Can you work these out from the drawing? Everything is in mm from the part's minimum corner. A direction names the side the tool comes from. Coordinates: 2 decimals unless noted, no trailing zeros. Loops run counter-clockwise (first coordinate to the right, second up) from the corner with the lowest first, then second, coordinate; pieces in that order, holes last. Notation, with made-up numbers: (50.25, -4.5) - (102.25, -4.5) arc R22 cw to (102.25, 25.5) - close; hole circle Ø10 at (55.5, 17). An arc over 180 degrees is marked (long way). Put each result on its own line as item: value. Start each with the question number.
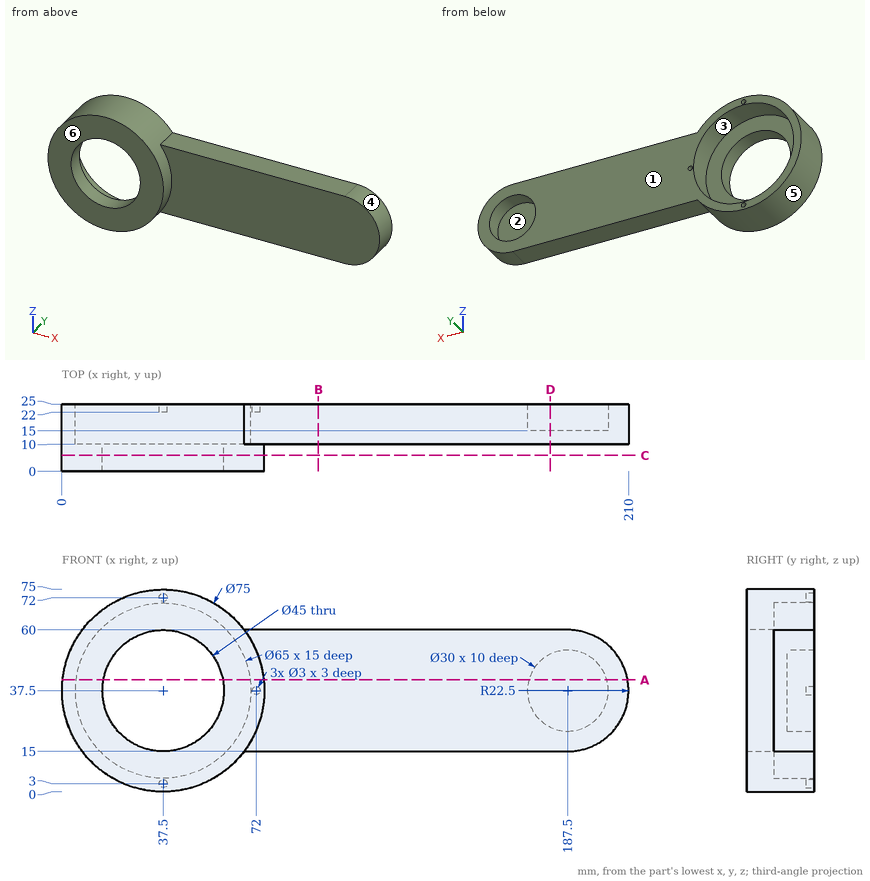
Q1. I want a section at C-C on y = 6. List the corners of the cut face in (x, z) for me, and give its area (3 significant figures).
Q2. Will these pins go through, and if not, where does the flat tip stop? pin 1 (2.5 mm diameter, centred on x = 37.5, z = 2.5, fed in from +Y); pin 2 (15 mm diameter, centred on x = 183.5, z = 40.5, fed in from +Y); pin 3 (8 mm diameter, centred on x = 141.5, y = 13, fed in from -Z); pin 4 (8 mm diameter, centred on x = 90.5, y = 17.5, fed in from +Z).
Q3. On a 3-axis mill with a long thin cutter (end or side, diameter ignored), from which of +Z, -Z, +X, -X, +Y, -Y can I reach the whole of each face in a straight line? I mean the marked faces 1 and 2. Say none if no direction works.
Q4. We'd pull the mould along X, two halves only. Please class the marked faces 3, 4, 5 and 6: released by +X, released by -X, zero draft, split by the parting line, or undercut.
Q5. Please list where these lines run through material, in increasing order: line 1 along X through (y, z) = (21, 37.5); line 2 along Z through (x, y) = (72, 23.3); line 3 along X through (y, z) = (17.5, 26.5). Write a range as [from, to].
Q6. I want a section at A-A on z = 41.5. List the corners of the cut face in (x, y) for me.
Q7. I want a section at B-B on x = 95. List the corners of the cut face in (y, z) for me, and give its area (3 significant figures).
Q8. I want a section at D-D on x = 181. List the corners of the cut face in (y, z) for me, and give its area (3 significant figures).
Calculated:
1. outline: circle Ø75 at (37.5, 37.5); hole circle Ø45 at (37.5, 37.5)
1. area: 2,830 mm2
2. pin 1: y = 25
2. pin 2: y = 15
2. pin 3: z = 15
2. pin 4: z = 60
3. face 1: +Z, -Z, +X, -X, +Y
3. face 2: +Y
4. face 3: undercut
4. face 4: released by +X
4. face 5: split by the parting line
4. face 6: zero draft
5. line 1: [0, 5], [70, 172.5], [202.5, 210]
5. line 2: [15, 36], [39, 60]
5. line 3: [1.65, 6.92], [68.08, 177.3], [197.7, 207.13]
6. outline: (0.21, 0) - (15.36, 0) - (15.36, 10) - (5.25, 10) - (5.25, 25) - (0.21, 25) - close; (59.64, 0) - (74.79, 0) - (74.79, 10) - (209.64, 10) - (209.64, 25) - (201.96, 25) - (201.96, 15) - (173.04, 15) - (173.04, 25) - (69.75, 25) - (69.75, 10) - (59.64, 10) - close
7. outline: (10, 15) - (25, 15) - (25, 60) - (10, 60) - close
7. area: 675 mm2
8. outline: (10, 15) - (25, 15) - (25, 23.98) - (15, 23.98) - (15, 51.02) - (25, 51.02) - (25, 60) - (10, 60) - close
8. area: 405 mm2
